Verification items for the finished model (mm, model axes). A direction names the side the tool comes from. Coordinates: 2 decimals unless noted, no trailing zeros. Loops run counter-clockwise (first coordinate to the right, second up) from the corner with the lowest first, then second, coordinate; pieces in that order, holes last.
Q1. Material ranges on probe 1 along X at (y, z) = (9.5, 0); probe 2 along Z at (x, y) = (-2, 2.25); probe 3 along Y at (x, z) = (6.5, 1.5), recorded low to high.
Q2. Sectioned sample at B-B (y = 11.25). Enter the section's corners in (x, z).
Q3. Access from +Z, -Z, +X, -X, +Y, -Y to the whole of each face (thin tool, end or side, straight path). Record for faces 1 (the face through (11.21, 11.13, 4.16)), 2 (the face through (13, 20, 0)).
Q4. Go/stop test with flat-tipped pins: P1, Ø5, axis at y = 16, z = 10.5, coming from the -X side; P2, Ø2, axis at x = -2, z = 7.25, coming from the +Y side; P3, Ø12, axis at y = 17.5, z = 13, coming from the -X side; P4, Ø1.5, axis at y = 17.5, z = 7, coming from the -X side. Record where each tip stops, or that it passes through.
Q5. Sectioned sample at A-A (z = 0). Enter the section's corners in (x, y).
Q6. Sectioned sample at C-C (x = -2.5). Count the separate pieces of the cut face and the enclosed holes in it, then the cut area to 3 significant figures.
Q7. Mould release check, pull along X, two halves, no side actions. Record for faces 3 (the face through (4, 3, 0)), 4 (the face through (4, 0, 0)), 5 (the face through (-2.343, 9.867, 17.847)): +X half, -X half, draft (parallel to the pull), parting line (faces both ways), or undercut.
Autodesk Fusion 360 part; units mm, degrees
sketch "スケッチ1" plane through (0, 0, 0) normal (0, 1, 0) x (1, 0, 0)
  circle A0 centre (0, 0) radius 18
  circle A1 centre (-2, 0) radius 13.85
  dimension "d5" = 27.7
extrude "押し出し2" add sketch "スケッチ1" along normal blind 20
sketch "スケッチ2" plane through (0, 0, 0) normal (0, 1, 0) x (1, 0, 0)
  circle A0 centre (-2, 0) radius 13.85
  circle A1 centre (-2, 0) radius 5
  dimension "d8" = 27.7
  dimension "d11" = 10
extrude "押し出し4" add sketch "スケッチ2" along normal blind 3
sketch "スケッチ3" plane through (0, 0, 0) normal (0, -1, 0) x (1, 0, 0)
  circle A0 centre (-2, 0) radius 5
  circle A1 centre (0, 0) radius 18
  circle A2 centre (-2, -7.25) radius 1.25
  line L0 (-2, 0) -> (-2, 7.25)
  circle A3 centre (-2, 7.25) radius 1.25
  point P0 (-2, 0)
  dimension "d14" = 7.25
  dimension "d15" = 2.5
  dimension "d16" = 7.25
  dimension "d17" = 2.5
extrude "押し出し5" cut sketch "スケッチ3" against normal blind 3 contours A3 | A2
chamfer "面取り1" distance 0.5 angle 45 2 edges at (-16.7819, 0, 6.5091) (-6.6616, 0, -1.8081)
chamfer "面取り2" distance 0.5 angle 45 2 edges at (-16.7819, 20, 6.5091) (-14.9127, 20, -5.0084)
sketch "スケッチ4" plane through (0, 0, 0) normal (0, 1, 0) x (1, 0, 0)
Geometry check:
1. probe 1: x = -18 to -15.85, 11.85 to 18
1. probe 2: z = -17.89 to -8.5, -6 to -5, 5 to 6, 8.5 to 17.89
1. probe 3: y = 0 to 3
2. outline: circle Ø36 at (0, 0); hole circle Ø27.7 at (-2, 0)
3. face 1: +Y
3. face 2: +Z, -Z, +X, -X, +Y
4. P1: stops at x = -16.12
4. P2: passes through
4. P3: stops at x = -16.58
4. P4: stops at x = -16.88
5. outline: (-18, 0.5) - (-17.5, 0) - (-7.5, 0) - (-7, 0.5) - (-7, 3) - (-15.85, 3) - (-15.85, 19.5) - (-16.35, 20) - (-17.5, 20) - (-18, 19.5) - close; (3, 0.5) - (3.5, 0) - (17.5, 0) - (18, 0.5) - (18, 19.5) - (17.5, 20) - (12.35, 20) - (11.85, 19.5) - (11.85, 3) - (3, 3) - close
6. separate pieces: 4
6. enclosed holes: 0
6. area: 198 mm2
7. face 3: undercut
7. face 4: draft
7. face 5: parting line
